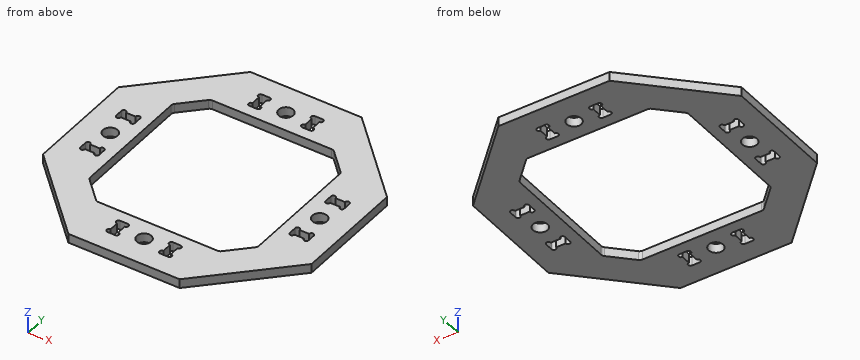
from build123d import *

# Parameters (mm, degrees)
SKETCH1_R           = 1.6
SKETCH1_W           = 4.1
SKETCH1_H           = 1.7
SKETCH1_W_2         = 1.7
SKETCH1_H_2         = 4.1
BOSS_EXTRUDE1_DEPTH = 2
CUT_EXTRUDE1_REACH  = 43.767
FILLET2_R           = 1
SKETCH4_R           = 0.5
CUT_EXTRUDE3_DEPTH  = 2


with BuildPart() as part:
    # Sketch1 → Boss-Extrude1 (new body)
    with BuildSketch(Plane.XY):
        Polygon((29.5, 12.21930009), (12.21930009, 29.5), (-12.21930009, 29.5), (-29.5, 12.21930009), (-29.5, -12.21930009), (-12.21930009, -29.5), (12.21930009, -29.5), (29.5, -12.21930009), align=None)
        with Locations((-23, 0)):
            Circle(SKETCH1_R, mode=Mode.SUBTRACT)
        with Locations((0, 23)):
            Circle(SKETCH1_R, mode=Mode.SUBTRACT)
        with Locations((23, 0)):
            Circle(SKETCH1_R, mode=Mode.SUBTRACT)
        with Locations((0, -23)):
            Circle(SKETCH1_R, mode=Mode.SUBTRACT)
        with Locations((-23, -5.8)):
            Rectangle(SKETCH1_W, SKETCH1_H, mode=Mode.SUBTRACT)
        with Locations((-5.8, 23)):
            Rectangle(SKETCH1_W_2, SKETCH1_H_2, mode=Mode.SUBTRACT)
        with Locations((-23, 5.8)):
            Rectangle(SKETCH1_W, SKETCH1_H, mode=Mode.SUBTRACT)
        with Locations((5.8, 23)):
            Rectangle(SKETCH1_W_2, SKETCH1_H_2, mode=Mode.SUBTRACT)
        with Locations((23, 5.8)):
            Rectangle(SKETCH1_W, SKETCH1_H, mode=Mode.SUBTRACT)
        with Locations((23, -5.8)):
            Rectangle(SKETCH1_W, SKETCH1_H, mode=Mode.SUBTRACT)
        with Locations((5.8, -23)):
            Rectangle(SKETCH1_W_2, SKETCH1_H_2, mode=Mode.SUBTRACT)
        with Locations((-5.8, -23)):
            Rectangle(SKETCH1_W_2, SKETCH1_H_2, mode=Mode.SUBTRACT)
    extrude(amount=-BOSS_EXTRUDE1_DEPTH)

    # Sketch2 → Cut-Extrude1 (cut, up to next)
    with BuildSketch(Plane(origin=(0, 0, 0), x_dir=(-1, 0, 0), z_dir=(0, 0, -1)), mode=Mode.PRIVATE) as cut_extrude1_sk1:
        Polygon((18.5, 13.5), (16, 16), (-16, -16), (-13.5, -18.5), (13.5, -18.5), (18.5, -13.5), align=None)
    cut_extrude1_tool1 = extrude(cut_extrude1_sk1.sketch, amount=CUT_EXTRUDE1_REACH, mode=Mode.PRIVATE) & part.part
    # Sketch2 → Cut-Extrude1 (cut, up to next)
    with BuildSketch(Plane(origin=(0, 0, 0), x_dir=(-1, 0, 0), z_dir=(0, 0, -1)), mode=Mode.PRIVATE) as cut_extrude1_sk2:
        Polygon((-16, -16), (16, 16), (13.5, 18.5), (-13.5, 18.5), (-18.5, 13.5), (-18.5, -13.5), align=None)
    cut_extrude1_tool2 = extrude(cut_extrude1_sk2.sketch, amount=CUT_EXTRUDE1_REACH, mode=Mode.PRIVATE) & part.part
    add(cut_extrude1_tool1.solids().sort_by_distance((-6.06558, -6.06558, 0))[0], mode=Mode.SUBTRACT)
    add(cut_extrude1_tool2.solids().sort_by_distance((6.06558, 6.06558, 0))[0], mode=Mode.SUBTRACT)

    # Fillet2
    fillet2_edges = [part.edges().sort_by_distance(p)[0] for p in [
        (18.5, -13.5, -1),
        (13.5, -18.5, -1),
        (-13.5, -18.5, -1),
        (-18.5, -13.5, -1),
        (-18.5, 13.5, -1),
        (-13.5, 18.5, -1),
        (13.5, 18.5, -1),
        (18.5, 13.5, -1),
    ]]
    fillet(fillet2_edges, radius=FILLET2_R)

    # Sketch4 → Cut-Extrude3 (cut)
    with BuildSketch(Plane.XY):
        with Locations((-24.55, 6.65)):
            Circle(SKETCH4_R)
        with Locations((-21.45, 6.65)):
            Circle(SKETCH4_R)
        with Locations((-21.45, 4.95)):
            Circle(SKETCH4_R)
        with Locations((-24.55, 4.95)):
            Circle(SKETCH4_R)
        with Locations((-24.55, -4.95)):
            Circle(SKETCH4_R)
        with Locations((-24.55, -6.65)):
            Circle(SKETCH4_R)
        with Locations((-21.45, -4.95)):
            Circle(SKETCH4_R)
        with Locations((-21.45, -6.65)):
            Circle(SKETCH4_R)
        with Locations((6.65, 21.45)):
            Circle(SKETCH4_R)
        with Locations((4.95, 21.45)):
            Circle(SKETCH4_R)
        with Locations((4.95, 24.55)):
            Circle(SKETCH4_R)
        with Locations((-4.95, 24.55)):
            Circle(SKETCH4_R)
        with Locations((-6.65, 24.55)):
            Circle(SKETCH4_R)
        with Locations((-4.95, 21.45)):
            Circle(SKETCH4_R)
        with Locations((-6.65, 21.45)):
            Circle(SKETCH4_R)
        with Locations((21.45, -6.65)):
            Circle(SKETCH4_R)
        with Locations((21.45, -4.95)):
            Circle(SKETCH4_R)
        with Locations((24.55, -4.95)):
            Circle(SKETCH4_R)
        with Locations((24.55, 4.95)):
            Circle(SKETCH4_R)
        with Locations((24.55, 6.65)):
            Circle(SKETCH4_R)
        with Locations((21.45, 4.95)):
            Circle(SKETCH4_R)
        with Locations((21.45, 6.65)):
            Circle(SKETCH4_R)
        with Locations((-6.65, -21.45)):
            Circle(SKETCH4_R)
        with Locations((-4.95, -21.45)):
            Circle(SKETCH4_R)
        with Locations((-4.95, -24.55)):
            Circle(SKETCH4_R)
        with Locations((4.95, -24.55)):
            Circle(SKETCH4_R)
        with Locations((6.65, -24.55)):
            Circle(SKETCH4_R)
        with Locations((4.95, -21.45)):
            Circle(SKETCH4_R)
        with Locations((6.65, -21.45)):
            Circle(SKETCH4_R)
        with Locations((6.65, 24.55)):
            Circle(SKETCH4_R)
        with Locations((24.55, -6.65)):
            Circle(SKETCH4_R)
        with Locations((-6.65, -24.55)):
            Circle(SKETCH4_R)
    extrude(amount=-CUT_EXTRUDE3_DEPTH, mode=Mode.SUBTRACT)


solid = part.part
Here's how the part is built. I have some questions about the finished solid (model axes, mm). Coordinates: 2 decimals unless noted, no trailing zeros. Order: outer loops, then holes, each group sorted by start corner. A loop starts at its lowest first (then second) coordinate and runs counter-clockwise, first axis right, second up. Notation, with made-up numbers: M 34.5,3 L 46.5,3 A24 ccw 46.5,36 Z; hole C 75,51 d9. An arc over 180 degrees is marked long. Answer as CSV lines item,"result". Start each with the question number.
1. I want a section at A-A, the plane x = 0. Write out the boundary of the cut face in (y, z), and give its area (3 significant figures).
2. I need wall thicknesses on line 1 (Y direction, x = 0, z = -1.6); line 2 (Y direction, x = -5.5, z = -0.65); line 3 (X direction, y = 10.5, z = -1.6). Which ranges of each line are inside material? Lowest first, please. Write a range as [from, to].
3. I want a section at C-C, the plane x = 10.5. Write out the boundary of the cut face in (y, z), and give its area (3 significant figures).
4. For pin 1 (1 mm diameter, centred on y = -23, z = -0.5, fed in from -X), with a flat end and sliding along its axis, tell me the tip position at first contact or that it passes through.
5. I want a section at D-D, the plane z = -0.7. Count the separate pieces of the cut face and the enclosed holes in it, and give its area (3 significant figures).
Recorded:
1,outline,"M -29.5,-2 L -24.6,-2 L -24.6,0 L -29.5,0 Z; M -21.4,-2 L -18.5,-2 L -18.5,0 L -21.4,0 Z; M 18.5,-2 L 21.4,-2 L 21.4,0 L 18.5,0 Z; M 24.6,-2 L 29.5,-2 L 29.5,0 L 24.6,0 Z"
1,area,"31.2 mm2"
2,line 1,"y = [-29.5, -24.6], [-21.4, -18.5], [18.5, 21.4], [24.6, 29.5]"
2,line 2,"y = [-29.5, -25.05], [-20.95, -18.5], [18.5, 20.95], [25.05, 29.5]"
2,line 3,"x = [-29.5, -18.5], [18.5, 29.5]"
3,outline,"M -29.5,-2 L -18.5,-2 L -18.5,0 L -29.5,0 Z; M 18.5,-2 L 29.5,-2 L 29.5,0 L 18.5,0 Z"
3,area,"44.0 mm2"
4,pin 1,"stops at x = -19.22"
5,separate pieces,"1"
5,enclosed holes,"13"
5,area,"1,460 mm2"
